Study the drawing (mm; zero at the part's minimum x, y, z) and answer. Give positions to 0.01 mm unless a question says otherwise; leave off trailing zeros. Loops run counter-clockwise (first coordinate to the right, second up) from the corner with the lowest first, then second, coordinate; pieces in that order, holes last. Notation, with made-up numbers: M 59.25,85.25 L 105.25,85.25 A20 cw 105.25,115.25 Z; hole C 38.25,-7.75 d4. An arc over 180 degrees is marked long. Use one line per item in the form item = value. Start each with the question number.
1. The part is cut by section C-C (x = 32). Write down the section's boundary in (y, z), and give its area (3 significant figures).
2. The part is cut by section A-A (z = 34.5). Write down the section's boundary in (x, y).
3. This flat-tipped pin is pushed along its axis until it touches: pin 1 Ø1.5 at (x, y) = (47.5, 2.5) entering from +Z. Where does it stop, or does it pass through?
4. The part is cut by section B-B (y = 1.7). Write down the section's boundary in (x, z), and give its area (3 significant figures).
5. Straight lines are drawn through the part: line 1 (Z direction, x = 18.5, y = 1.4) (1 decimal); line 2 (Z direction, x = 30, y = 0.55) (1 decimal); line 3 (X direction, y = 2.85, z = 75) (1 decimal). For each, find the intervals that lie inside material, in ascending order. Write a range as from..to.
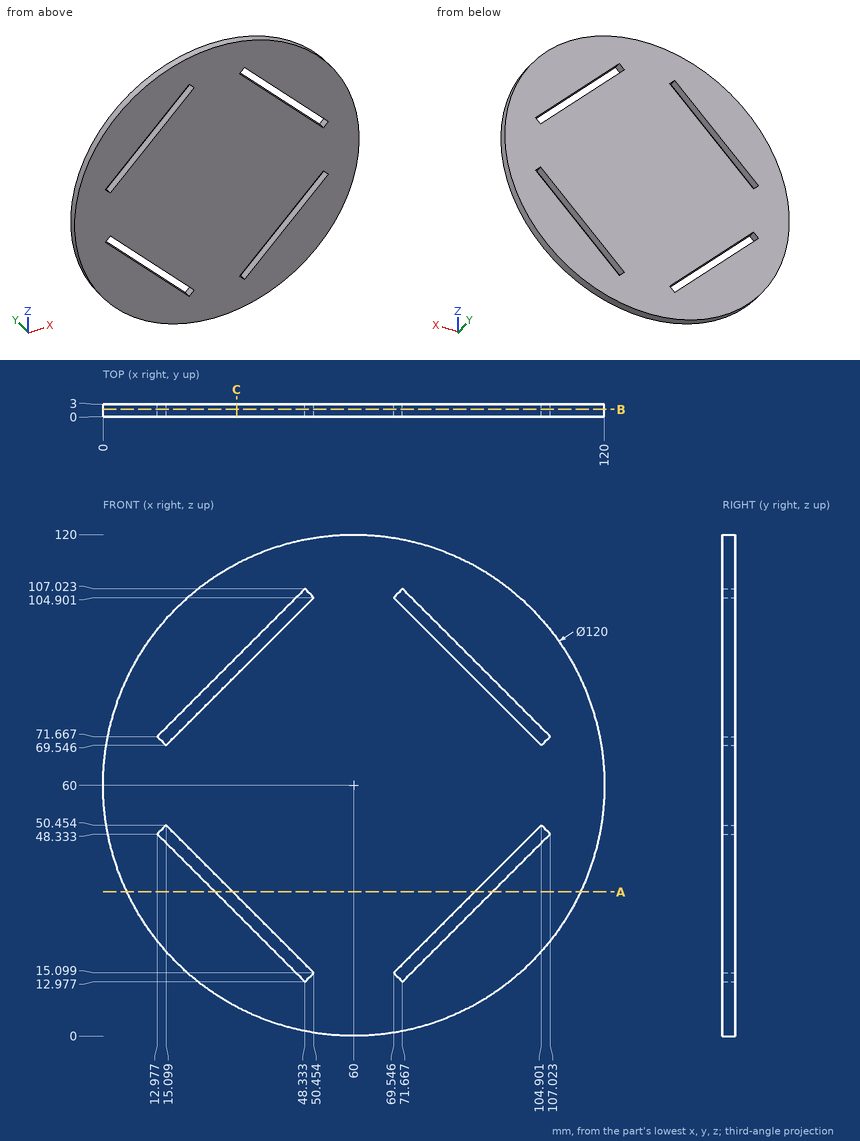
Derived:
q1.outline = M 0,6.93 L 3,6.93 L 3,29.31 L 0,29.31 Z; M 0,33.55 L 3,33.55 L 3,86.45 L 0,86.45 Z; M 0,90.69 L 3,90.69 L 3,113.07 L 0,113.07 Z
q1.area = 293 mm2
q2.outline = M 5.69,0 L 26.81,0 L 26.81,3 L 5.69,3 Z; M 31.05,0 L 88.95,0 L 88.95,3 L 31.05,3 Z; M 93.19,0 L 114.31,0 L 114.31,3 L 93.19,3 Z
q3.pin_1 = 118.84
q4.outline = C 60,60 d120; hole M 12.98,48.33 L 48.33,12.98 L 50.45,15.1 L 15.1,50.45 Z; hole M 12.98,71.67 L 15.1,69.55 L 50.45,104.9 L 48.33,107.02 Z; hole M 69.55,15.1 L 71.67,12.98 L 107.02,48.33 L 104.9,50.45 Z; hole M 69.55,104.9 L 104.9,69.55 L 107.02,71.67 L 71.67,107.02 Z
q4.area = 10,700 mm2
q5.line_1 = 16.7..42.8, 47.1..72.9, 77.2..103.3
q5.line_2 = 8..31.3, 35.6..84.4, 88.7..112
q5.line_3 = 1.9..16.3, 20.6..99.4, 103.7..118.1
